Autodesk Inventor part; units mm, degrees
ref_plane "YZ Plane" through (0, 0, 0) normal (1, 0, 0) x (0, 1, 0)
ref_plane "XZ Plane" through (0, 0, 0) normal (0, 1, 0) x (-1, 0, 0)
ref_plane "XY Plane" through (0, 0, 0) normal (0, 0, 1) x (1, 0, 0)
sketch "Sketch1" plane through (0, 0, 0) normal (0, 0, 1) x (1, 0, 0)
  line L0 (-2.2451, -2.2451) -> (-26.9408, -26.9408)
  line L1 (2.2451, -2.2451) -> (26.9408, -26.9408)
  line L2 (2.2451, 2.2451) -> (26.9408, 26.9408)
  line L3 (-2.2451, 2.2451) -> (-26.9408, 26.9408)
  circle A0 centre (0, 0) radius 1.5875
  arc A1 (2.2451, -2.2451) -> (2.2451, 2.2451) centre (0, 0) ccw
  arc A2 (-2.2451, 2.2451) -> (-2.2451, -2.2451) centre (0, 0) ccw
  line L4 (0, 0) -> (-1.5875, 0)
  arc A3 (26.9408, 26.9408) -> (-26.9408, 26.9408) centre (0, 0) ccw
  arc A4 (-26.9408, -26.9408) -> (26.9408, -26.9408) centre (0, 0) ccw
  dimension "d5" = 3.175
  dimension "d1" = 90
  dimension "d2" = 90
  dimension "d3" = 90
extrude "Extrusion1" add sketch "Sketch1" along normal blind 3.175
properties part number "Release2"
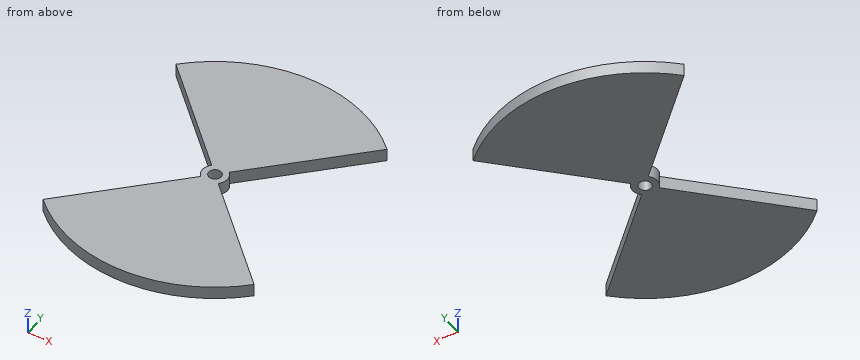
The listing builds one solid part. Answer for the finished solid, in the listing's coordinates (mm). Coordinates: 2 decimals unless noted, no trailing zeros. Loops run counter-clockwise (first coordinate to the right, second up) from the corner with the lowest first, then second, coordinate; pieces in that order, holes last. Notation, with made-up numbers: (64.5, 25) -> (77.5, 25) arc R28 ccw to (77.5, 45) -> close; hole circle Ø2 at (64.25, -20.75). An arc over 180 degrees is marked (long way). Answer in a Markdown table with one row per item. Add a question column.
1. Consider line 1 (Y direction, x = 0, z = 0.85); line 2 (X direction, y = 0, z = 1); line 3 (Y direction, x = 6.5, z = 2.8). Determine where each line is inside the solid, lowest interval first. Write a range as [from, to].
2. The part is cut by section D-D, the plane y = 8. Write down the section's boundary in (x, z) (3 decimals), then the cut area to 3 significant figures.
3. The part is cut by section A-A, the plane x = 0. Write down the section's boundary in (y, z) (1 decimal).
4. The part is cut by section B-B, the plane y = 0. Write down the section's boundary in (x, z) (1 decimal).
5. Flat-ended cylindrical pins translate along their axes: P1, Ø2.5, axis at x = 0, y = 0, coming from the -Z side; P2, Ø1.5, axis at x = 1, z = 2.5, coming from the -Y side. Find the tip coordinate at first contact, or state that the pin passes through.
6. The part is cut by section C-C, the plane z = 2.4. Write down the section's boundary in (x, y) (1 decimal), then the cut area to 3 significant figures.
Answer below:
| question | item | result |
|---|---|---|
| 1 | line 1 | [-38.1, -1.59], [1.59, 38.1] |
| 1 | line 2 | [-3.18, -1.59], [1.59, 3.18] |
| 1 | line 3 | [-37.54, -6.5], [6.5, 37.54] |
| 2 | outline | (-8, 0) -> (8, 0) -> (8, 3.175) -> (-8, 3.175) -> close |
| 2 | area | 50.8 mm2 |
| 3 | outline | (-38.1, 0) -> (-1.6, 0) -> (-1.6, 3.2) -> (-38.1, 3.2) -> close; (1.6, 0) -> (38.1, 0) -> (38.1, 3.2) -> (1.6, 3.2) -> close |
| 4 | outline | (-3.2, 0) -> (-1.6, 0) -> (-1.6, 3.2) -> (-3.2, 3.2) -> close; (1.6, 0) -> (3.2, 0) -> (3.2, 3.2) -> (1.6, 3.2) -> close |
| 5 | P1 | through |
| 5 | P2 | y = -38.1 |
| 6 | outline | (-26.9, -26.9) arc R38.1 ccw to (26.9, -26.9) -> (2.2, -2.2) arc R3.2 ccw to (2.2, 2.2) -> (26.9, 26.9) arc R38.1 ccw to (-26.9, 26.9) -> (-2.2, 2.2) arc R3.2 ccw to (-2.2, -2.2) -> close; hole circle Ø3.2 at (0, 0) |
| 6 | area | 2,290 mm2 |
